Source: three-view drawing plus pictorial views. Frame: mm from the lowest corner of the part. A direction names the side the tool comes from. Round coordinates to 2 decimals unless told otherwise and drop trailing zeros. Write each loop counter-clockwise with the first axis right and the second up, starting at its lowest first coordinate (ties: lowest second). Pieces come first, ordered by that corner, then holes. Notation, with made-up numbers: (23, 34.5) -> (54, 34.5) arc R19 ccw to (54, 63.5) -> close; hole circle Ø10 at (-24.5, 33.5). An arc over 180 degrees is marked (long way). Put each result on its own line as item: value.
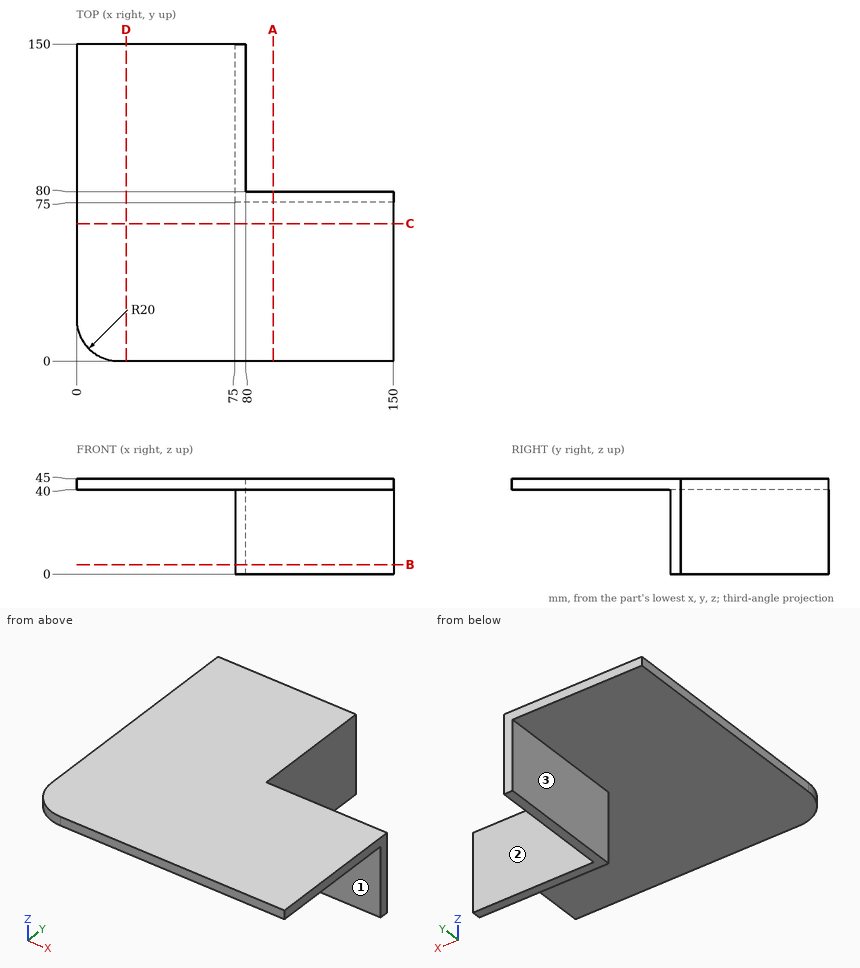
Q1. Material intervals for line 1 (Z direction, x = 25.5, y = 19); line 2 (X direction, y = 78, z = 13); line 3 (X direction, y = 117.5, z = 15), sorted ascending. Write a range as [from, to].
Ans:
line 1: z = [40, 45]
line 2: x = [75, 150]
line 3: x = [75, 80]
Q2. Reachability of the marked faces 1, 2 and 3 from +Z, -Z, +X, -X, +Y, -Y: full face, straight path, thin tool, end or side. Return the list, or none.
Ans:
face 1: -Z, +X, -X, -Y
face 2: +Z, -Z, +X, +Y
face 3: -Z, -X, +Y, -Y
Q3. Cut plane A-A on x = 93. Output: boundary loops of the cut face in (y, z), and give its area (3 significant figures).
Ans:
outline: (0, 40) -> (75, 40) -> (75, 0) -> (80, 0) -> (80, 45) -> (0, 45) -> close
area: 600 mm^2
Q4. Cut plane B-B on z = 4.5. Output: boundary loops of the cut face in (x, y).
Ans:
outline: (75, 75) -> (150, 75) -> (150, 80) -> (80, 80) -> (80, 150) -> (75, 150) -> close
Q5. Pin query (flat end, axial travel): pin 1 (8 mm diameter, centred on x = 129, z = 6.5, fed in from -Y); pin 2 (6 mm diameter, centred on x = 18.5, y = 96.5, fed in from -Z); pin 3 (13.5 mm diameter, centred on y = 118, z = 33.5, fed in from +X). Return the tip coordinate at first contact, or that it passes through.
Ans:
pin 1: stops at y = 75
pin 2: stops at z = 40
pin 3: stops at x = 80
Q6. Cut plane C-C on y = 65. Output: boundary loops of the cut face in (x, z).
Ans:
outline: (0, 40) -> (150, 40) -> (150, 45) -> (0, 45) -> close
